```python
from build123d import *

# Parameters (mm, degrees)
F1_DEPTH = 2.032


with BuildPart() as f1:
    # F0 (on Top) → F1 (new body)
    with BuildSketch(Plane.XY):
        with BuildLine():
            ThreePointArc((-18.497407, 6.858), (-15.73527, 3.911855), (-14.732, 0))
            ThreePointArc((-14.732, 0), (-15.73527, -3.911855), (-18.497407, -6.858))
            Line((-18.497407, -6.858), (18.497407, -6.858))
            ThreePointArc((18.497407, -6.858), (14.732, 0), (18.497407, 6.858))
            Line((18.497407, 6.858), (-18.497407, 6.858))
        make_face()
    extrude(amount=F1_DEPTH)

    # F2 (on Front) → F3 (revolve)
    with BuildSketch(Plane.XZ):
        Polygon((-32.258, 2.032), (-32.258, 0), (-30.226, 0), (-30.226, 0.508), (-30.734, 1.016), (-30.226, 1.524), (-30.226, 2.032), align=None)
    revolve(axis=Axis((-22.86, 0, 0.9144), (0, 0, 1)))

    # F4: F1 across plane


with BuildPart() as f1_1:
    add(f1.part)
    add(f1.part.mirror(Plane.YZ))


solid = f1_1.part
```
Part model, mm, in its own coordinate system. A direction names the side the tool comes from. Round coordinates to 2 decimals unless told otherwise and drop trailing zeros. Order: outer loops, then holes, each group sorted by start corner. A loop starts at its lowest first (then second) coordinate and runs counter-clockwise, first axis right, second up. Notation, with made-up numbers: M 0.5,15.25 L 31.5,15.25 A8 cw 31.5,24.25 Z; hole C 38.5,-3 d8. An arc over 180 degrees is marked long. Answer in a Markdown table with one row per item. Add a question column.
Q1. Cut at B-B on y = 0. Give the cut face in (x, z), and give its area (3 significant figures).
Q2. Pin check, flat tips, straight feed: pin 1 (1 mm diameter, centred on x = -12, z = 0.5, fed in from -Y); pin 2 (0.6 mm diameter, centred on x = 1.5, z = 1.5, fed in from +Y). Stop position of each tip, or through.
Q3. Mould opens along Y. For faces 1 (the face through (0, -6.858, 1)), 2 (the face through (-32.253, 0.306, 1.002)), 3 (the face through (0, 0, 2.032)), 4 (the face through (29.664, 2.821, 0.258)) say: +Y half, -Y half, draft (parallel to the pull), parting line (faces both ways), or undercut.
Q4. Wall check: L1, parallel to X at y = 0, z = 0.4; L2, parallel to Y at x = -22.86, z = 0.15; L3, parallel to X at y = -5, z = 1.55. Give the ranges that are in metal, low to high. Write a range as from..to.
Q5. Cut at D-D on y = -2.5. Give the number of separate pieces and of enclosed holes in the cut face, and give its area (3 significant figures).
Q6. 3-axis set-ups, long thin cutter, end or side, ignore diameter. For faces 5 (the face through (0, 6.858, 1)), 6 (the face through (-29.664, 2.821, 0.258)): which of +Z, -Z, +X, -X, +Y, -Y reach the whole face in a straight line?
Q7. Cut at C-C on x = -12. Give the cut face in (y, z).
Q8. Cut at A-A on x = 22.86. Give the cut face in (y, z), and give its area (3 significant figures).
Established:
| question | item | result |
|---|---|---|
| 1 | outline | M -32.26,0 L -30.23,0 L -30.23,0.51 L -30.73,1.02 L -30.23,1.52 L -30.23,2.03 L -32.26,2.03 Z; M -15.49,0 L 15.49,0 L 15.49,0.51 L 14.99,1.02 L 15.49,1.52 L 15.49,2.03 L -15.49,2.03 L -15.49,1.52 L -14.99,1.02 L -15.49,0.51 Z; M 30.23,0 L 32.26,0 L 32.26,2.03 L 30.23,2.03 L 30.23,1.52 L 30.73,1.02 L 30.23,0.51 Z |
| 1 | area | 70.2 mm2 |
| 2 | pin 1 | stops at y = -6.86 |
| 2 | pin 2 | stops at y = 6.86 |
| 3 | face 1 | -Y half |
| 3 | face 2 | parting line |
| 3 | face 3 | draft |
| 3 | face 4 | undercut |
| 4 | L1 | x = -32.26..-30.23, -15.49..15.49, 30.23..32.26 |
| 4 | L2 | y = -9.4..-7.37, 7.37..9.4 |
| 4 | L3 | x = -30.82..-28.27, -17.45..17.45, 28.27..30.82 |
| 5 | separate pieces | 3 |
| 5 | enclosed holes | 0 |
| 5 | area | 72.3 mm2 |
| 6 | face 5 | +Z, -Z, +Y |
| 6 | face 6 | +Z, -Z |
| 7 | outline | M -6.86,0 L 6.86,0 L 6.86,2.03 L -6.86,2.03 Z |
| 8 | outline | M -9.4,0 L -7.37,0 L -7.37,0.51 L -7.87,1.02 L -7.37,1.52 L -7.37,2.03 L -9.4,2.03 Z; M 7.37,0 L 9.4,0 L 9.4,2.03 L 7.37,2.03 L 7.37,1.52 L 7.87,1.02 L 7.37,0.51 Z |
| 8 | area | 7.74 mm2 |
